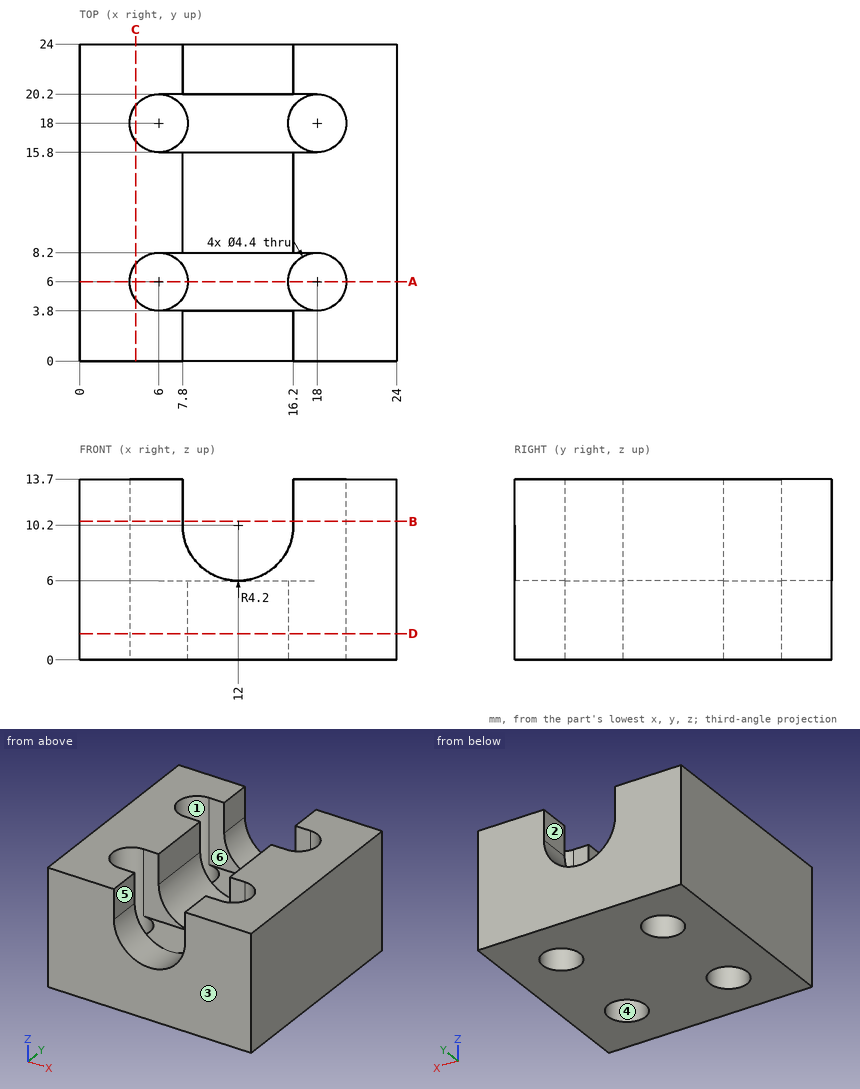
Part print with two shaded views. Sizes in mm from the minimum x, y, z corner. A direction names the side the tool comes from. Give positions to 0.01 mm unless a question says otherwise; leave off trailing zeros. Order: outer loops, then holes, each group sorted by start corner. A loop starts at its lowest first (then second) coordinate and runs counter-clockwise, first axis right, second up. Notation, with made-up numbers: M 75.25,24 L 109.25,24 A28 cw 109.25,58 Z; hole C 57.25,56 d11. An arc over 180 degrees is marked long. Put each result on its own line as item: value.
Item 1: Pull direction Y, two halves, no side cores. Call the marked faces 1, 2 and 3: +Y half, -Y half, draft (parallel to the pull), parting line (faces both ways), or undercut.
Results are:
face 1: undercut
face 2: draft
face 3: -Y half
Item 2: Wall check: probe 1 along Y at (x, z) = (6, 8.25); probe 2 along X at (y, z) = (21.25, 11.25); probe 3 along Y at (x, z) = (20, 6.75). Give the ranges that are in metal, low to high.
Results are:
probe 1: 0 to 3.8, 8.2 to 15.8, 20.2 to 24
probe 2: 0 to 7.8, 16.2 to 24
probe 3: 0 to 5.08, 6.92 to 17.08, 18.92 to 24
Item 3: Cut at A-A on y = 6. Write the cut outline in (x, z), then the cut area to 3 significant figures.
Results are:
outline: M 0,0 L 3.8,0 L 3.8,13.7 L 0,13.7 Z; M 8.2,0 L 15.8,0 L 15.8,6 L 8.2,6 Z; M 20.2,0 L 24,0 L 24,13.7 L 20.2,13.7 Z
area: 150 mm2
Item 4: Drop a flat-ended pin along its axis: pin 1 Ø1.3 at (x, y) = (13, 19) entering from +Z. Give the stop position or say it passes through.
Results are:
pin 1: z = 6
Item 5: Cut at D-D on z = 2. Write the cut outline in (x, y).
Results are:
outline: M 0,0 L 24,0 L 24,24 L 0,24 Z; hole C 6,6 d4.4; hole C 6,18 d4.4; hole C 18,6 d4.4; hole C 18,18 d4.4
Item 6: Which spindle directions (+Z, -Z, +X, -X, +Y, -Y) get a long thin tool onto all of the face, cutting with end or side? Do the marked faces 4, 5 and 6. Say none if no direction does.
Results are:
face 4: +Z, -Z
face 5: +Z, +Y, -Y
face 6: +Z
Item 7: Cut at B-B on z = 10.5. Write the cut outline in (x, y).
Results are:
outline: M 0,0 L 7.8,0 L 7.8,3.8 L 6,3.8 A2.2 cw 6,8.2 L 7.8,8.2 L 7.8,15.8 L 6,15.8 A2.2 cw 6,20.2 L 7.8,20.2 L 7.8,24 L 0,24 Z; M 16.2,0 L 24,0 L 24,24 L 16.2,24 L 16.2,20.2 L 18,20.2 A2.2 cw 18,15.8 L 16.2,15.8 L 16.2,8.2 L 18,8.2 A2.2 cw 18,3.8 L 16.2,3.8 Z
Item 8: Cut at C-C on x = 4.25. Write the cut outline in (y, z).
Results are:
outline: M 0,0 L 4.67,0 L 4.67,13.7 L 0,13.7 Z; M 7.33,0 L 16.67,0 L 16.67,13.7 L 7.33,13.7 Z; M 19.33,0 L 24,0 L 24,13.7 L 19.33,13.7 Z
